The figure shows three views and two pictorial views of one solid part (mm, origin at its lowest corner). Answer the questions. A direction names the side the tool comes from. Coordinates: 2 decimals unless noted, no trailing zeros. Order: outer loops, then holes, each group sorted by start corner. A loop starts at its lowest first (then second) coordinate and runs counter-clockwise, first axis right, second up. Notation, with made-up numbers: M -32,62.5 L 16,62.5 A21 cw 16,89.5 Z; hole C -23,76.25 d5. An arc over 180 degrees is marked long. Use a Markdown table: item, result.
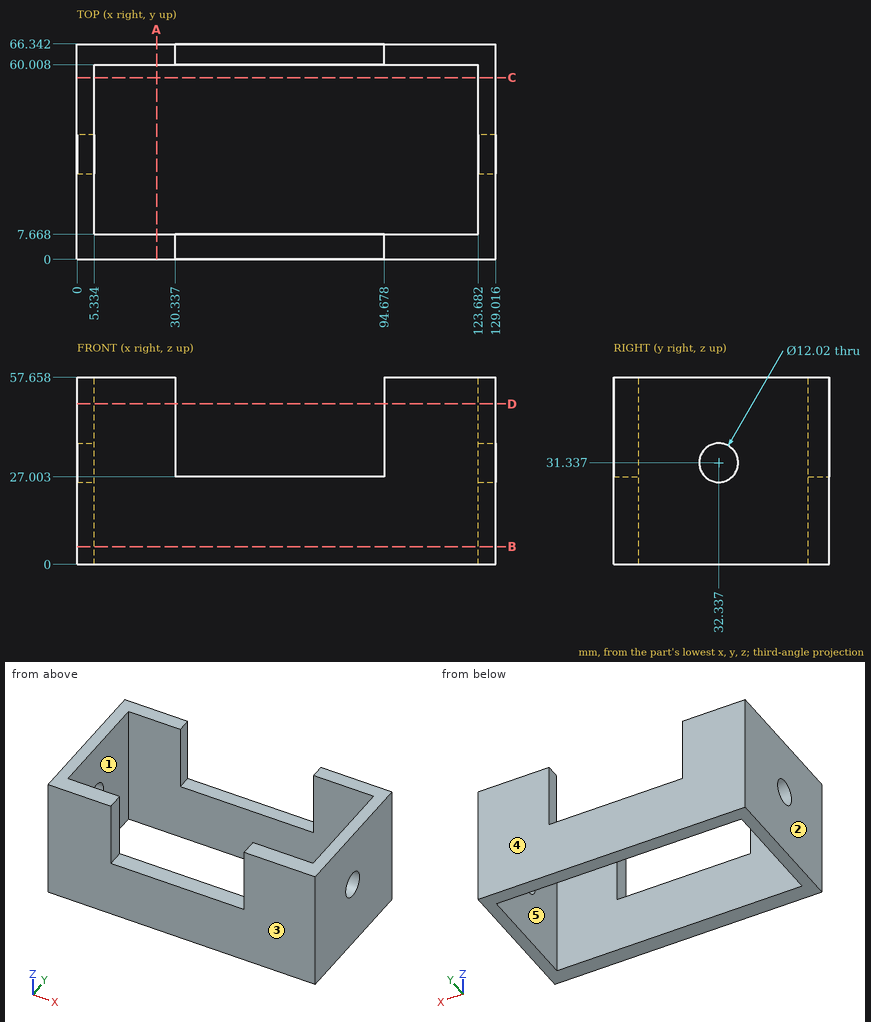
1. For the marked faces 1 and 2, determine the directions among +Z, -Z, +X, -X, +Y, -Y from which every point of the face is accessible in a straight line to the end or side of a thin tool.
Answers below:
| item | result |
|---|---|
| face 1 | +Z, -Z |
| face 2 | +Z, -Z, -X, +Y, -Y |
2. Section B-B on z = 5.5 is taken. Determine the outline of the cut face in (x, y) (1 decimal).
Answers below:
| item | result |
|---|---|
| outline | M 0,0 L 129,0 L 129,66.3 L 0,66.3 Z; hole M 5.3,7.7 L 123.7,7.7 L 123.7,60 L 5.3,60 Z |
3. Flat-ended cylindrical pins translate along their axes: P1, Ø11, axis at y = 32.34, z = 31.34, coming from the +X side; P2, Ø4, axis at x = 48, y = 4.5, coming from the +Z side. Find the tip coordinate at first contact, or state that the pin passes through.
Answers below:
| item | result |
|---|---|
| P1 | through |
| P2 | z = 27 |
4. Find the intervals of material crossed by probe 1 along X at (y, z) = (51, 27.5) (1 decimal); probe 2 along Y at (x, z) = (14.5, 46.5); probe 3 along Z at (x, y) = (85, 6), in increasing order.
Answers below:
| item | result |
|---|---|
| probe 1 | 0 to 5.3, 123.7 to 129 |
| probe 2 | 0 to 7.67, 60.01 to 66.34 |
| probe 3 | 0 to 27 |
5. Section A-A on x = 24.5 is taken. Determine the outline of the cut face in (y, z).
Answers below:
| item | result |
|---|---|
| outline | M 0,0 L 7.67,0 L 7.67,57.66 L 0,57.66 Z; M 60.01,0 L 66.34,0 L 66.34,57.66 L 60.01,57.66 Z |
6. For a pull along Y with two mould halves and no side action, classify the marked faces 3, 4 and 5 as +Y half, -Y half, draft (parallel to the pull), parting line (faces both ways), or undercut.
Answers below:
| item | result |
|---|---|
| face 3 | -Y half |
| face 4 | +Y half |
| face 5 | undercut |
7. Section C-C on y = 56 is taken. Determine the outline of the cut face in (x, z) (1 decimal), then the cut area to 3 significant figures.
Answers below:
| item | result |
|---|---|
| outline | M 0,0 L 5.3,0 L 5.3,57.7 L 0,57.7 Z; M 123.7,0 L 129,0 L 129,57.7 L 123.7,57.7 Z |
| area | 615 mm² |
8. Section D-D on z = 49.5 is taken. Determine the outline of the cut face in (x, y) (1 decimal).
Answers below:
| item | result |
|---|---|
| outline | M 0,0 L 30.3,0 L 30.3,7.7 L 5.3,7.7 L 5.3,60 L 30.3,60 L 30.3,66.3 L 0,66.3 Z; M 94.7,0 L 129,0 L 129,66.3 L 94.7,66.3 L 94.7,60 L 123.7,60 L 123.7,7.7 L 94.7,7.7 Z |
